Input: dimensioned drawing with shaded views. Units: mm. Origin: part minimum x, y, z. Coordinates: 2 decimals unless noted, no trailing zeros. Order: outer loops, then holes, each group sorted by start corner. A loop starts at its lowest first (then second) coordinate and runs counter-clockwise, first axis right, second up. Notation, with made-up numbers: M -17,-34.75 L 5,-34.75 A22 cw 5,-3.75 Z; hole C 59,24.25 d1. An arc over 180 degrees is marked long. Write item = value, one per line.
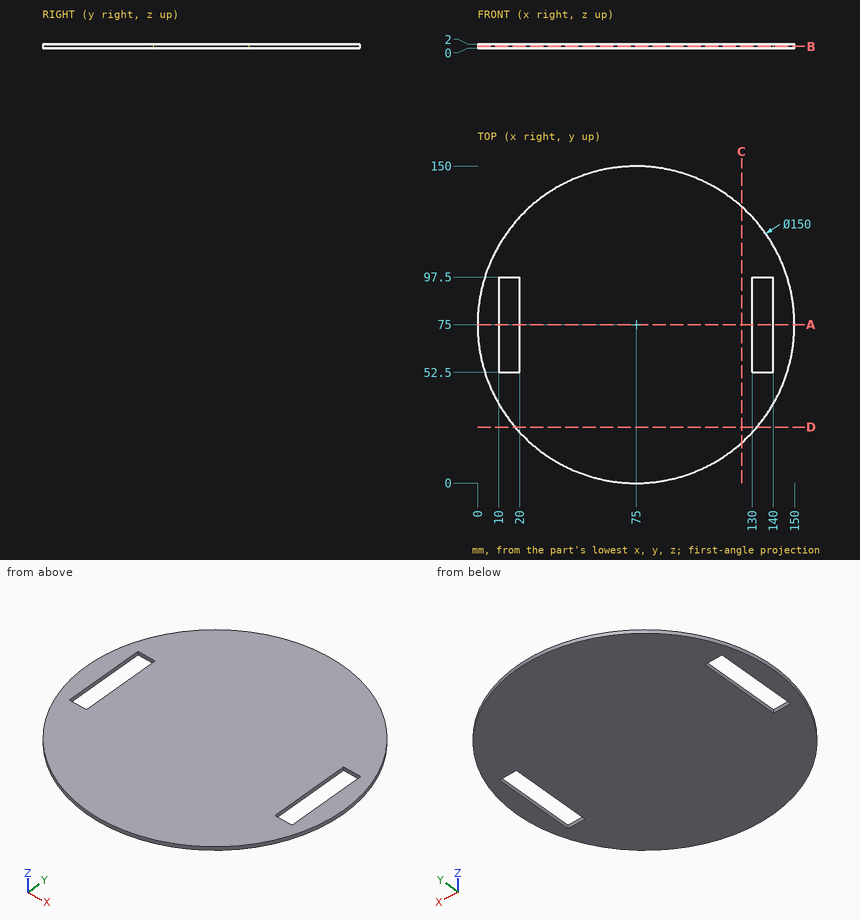
1) Section D-D, the plane y = 26.5. Return loops of the section in (x, z), and give its area (3 significant figures).
Numbers:
outline = M 17.79,0 L 132.21,0 L 132.21,2 L 17.79,2 Z
area = 229 mm²
2) Section A-A, the plane y = 75. Return loops of the section in (x, z).
Numbers:
outline = M 0,0 L 10,0 L 10,2 L 0,2 Z; M 20,0 L 130,0 L 130,2 L 20,2 Z; M 140,0 L 150,0 L 150,2 L 140,2 Z
3) Section C-C, the plane x = 125. Return loops of the section in (y, z), and give its area (3 significant figures).
Numbers:
outline = M 19.1,0 L 130.9,0 L 130.9,2 L 19.1,2 Z
area = 224 mm²
4) Section B-B, the plane z = 0.85. Return loops of the section in (x, y).
Numbers:
outline = C 75,75 d150; hole M 10,52.5 L 20,52.5 L 20,97.5 L 10,97.5 Z; hole M 130,52.5 L 140,52.5 L 140,97.5 L 130,97.5 Z
5) Pin query (flat end, axial travel): pin 1 (1 mm diameter, centred on y = 86, z = 1, fed in from +X); pin 2 (0.6 mm diameter, centred on y = 77, z = 0.5, fed in from -X). Return the tip coordinate at first contact, or that it passes through.
Numbers:
pin_1 = 149.26
pin_2 = 0.02
6) Line query: L1, parallel to X at y = 73, z = 1.25; L2, parallel to X at y = 63.5, z = 0.8; L3, parallel to Y at x = 10.5, z = 0.5. Output: solid intervals per line, ascending.
Numbers:
L1 = 0.03 to 10, 20 to 130, 140 to 149.97
L2 = 0.89 to 10, 20 to 130, 140 to 149.11
L3 = 36.73 to 52.5, 97.5 to 113.27
